```python
from build123d import *
from OCP.BRepFilletAPI import BRepFilletAPI_MakeChamfer

# Parameters (mm, degrees)
BASE_PLATE_DEPTH         = 3
INNER_START              = -3
INNER_BASE_PROFILE_DEPTH = 4
MOUNTING_START           = -7
BASEPLATE_5_R            = 1.83
MOUNTING_HOLES_DEPTH     = 7
COUNTERSINK_SIZE         = 1.7
COUNTERSINK_SIZE2        = 1.477787454


with BuildPart() as part:
    # BasePlate → Base Plate (new body)
    with BuildSketch(Plane(origin=(0, 0, 0), x_dir=(1, 0, 0), z_dir=(0, 1, 0))):
        with BuildLine():
            Line((-85, 75), (85, 75))
            ThreePointArc((85, 75), (95.606601718, 70.606601718), (100, 60))
            Line((100, 60), (100, -60))
            ThreePointArc((100, -60), (95.606601718, -70.606601718), (85, -75))
            Line((85, -75), (-85, -75))
            ThreePointArc((-85, -75), (-95.606601718, -70.606601718), (-100, -60))
            Line((-100, -60), (-100, 60))
            ThreePointArc((-100, 60), (-95.606601718, 70.606601718), (-85, 75))
        make_face()
    extrude(amount=-BASE_PLATE_DEPTH)

    # BasePlate<4> → Inner Base Profile (add)
    with BuildSketch(Plane(origin=(0, 0, 0), x_dir=(1, 0, 0), z_dir=(0, 1, 0)).offset(INNER_START)):
        with BuildLine():
            Line((-85, 73), (46, 73))
            ThreePointArc((46, 73), (47.414213562, 72.414213562), (48, 71))
            ThreePointArc((48, 71), (50, 69), (52, 71))
            ThreePointArc((52, 71), (52.585786438, 72.414213562), (54, 73))
            Line((54, 73), (85, 73))
            ThreePointArc((85, 73), (94.192388155, 69.192388155), (98, 60))
            Line((98, 60), (98, -60))
            ThreePointArc((98, -60), (94.192388155, -69.192388155), (85, -73))
            Line((85, -73), (54, -73))
            ThreePointArc((54, -73), (52.585786438, -72.414213562), (52, -71))
            ThreePointArc((52, -71), (50, -69), (48, -71))
            ThreePointArc((48, -71), (47.414213562, -72.414213562), (46, -73))
            Line((46, -73), (-85, -73))
            ThreePointArc((-85, -73), (-94.192388155, -69.192388155), (-98, -60))
            Line((-98, -60), (-98, 60))
            ThreePointArc((-98, 60), (-94.192388155, 69.192388155), (-85, 73))
        make_face()
    extrude(amount=-INNER_BASE_PROFILE_DEPTH)

    # BasePlate<5> → Mounting Holes (cut)
    with BuildSketch(Plane(origin=(0, 0, 0), x_dir=(1, 0, 0), z_dir=(0, 1, 0)).offset(MOUNTING_START)):
        with Locations(Location((90, -15, 0), (0, 0, 270))):
            Circle(BASEPLATE_5_R)
        with Locations(Location((-89, 64, 0), (0, 0, 270))):
            Circle(BASEPLATE_5_R)
        with Locations(Location((89, 64, 0), (0, 0, 270))):
            Circle(BASEPLATE_5_R)
        with Locations(Location((89, -64, 0), (0, 0, 270))):
            Circle(BASEPLATE_5_R)
        with Locations(Location((-89, -64, 0), (0, 0, 270))):
            Circle(BASEPLATE_5_R)
        with Locations(Location((0, 65, 0), (0, 0, 270))):
            Circle(BASEPLATE_5_R)
        with Locations(Location((-90, 0, 0), (0, 0, 270))):
            Circle(BASEPLATE_5_R)
        with Locations(Location((0, -65, 0), (0, 0, 270))):
            Circle(BASEPLATE_5_R)
    extrude(amount=MOUNTING_HOLES_DEPTH, mode=Mode.SUBTRACT)

    # Countersink: one chamfer whose edges measure the first distance from different faces: ONE call of the kernel's chamfer builder (chamfer() names one face for all edges)
    countersink_edges_1 = [part.edges().sort_by_distance(p)[0] for p in [
        (-89, 0, 62.17),
    ]]
    countersink_side_1 = [part.faces().sort_by_distance(p)[0] for p in [
        (-89, -3.5, 62.17),
    ]]
    countersink_edges_2 = [part.edges().sort_by_distance(p)[0] for p in [
        (0, 0, -66.83),
    ]]
    countersink_side_2 = [part.faces().sort_by_distance(p)[0] for p in [
        (0, -3.5, -66.83),
    ]]
    countersink_edges_3 = [part.edges().sort_by_distance(p)[0] for p in [
        (89, 0, -65.83),
    ]]
    countersink_side_3 = [part.faces().sort_by_distance(p)[0] for p in [
        (89, -3.5, -65.83),
    ]]
    countersink_edges_4 = [part.edges().sort_by_distance(p)[0] for p in [
        (90, 0, 13.17),
    ]]
    countersink_side_4 = [part.faces().sort_by_distance(p)[0] for p in [
        (90, -3.5, 13.17),
    ]]
    countersink_edges_5 = [part.edges().sort_by_distance(p)[0] for p in [
        (89, 0, 62.17),
    ]]
    countersink_side_5 = [part.faces().sort_by_distance(p)[0] for p in [
        (89, -3.5, 62.17),
    ]]
    countersink_edges_6 = [part.edges().sort_by_distance(p)[0] for p in [
        (-90, 0, -1.83),
    ]]
    countersink_side_6 = [part.faces().sort_by_distance(p)[0] for p in [
        (-90, -3.5, -1.83),
    ]]
    countersink_edges_7 = [part.edges().sort_by_distance(p)[0] for p in [
        (-89, 0, -65.83),
    ]]
    countersink_side_7 = [part.faces().sort_by_distance(p)[0] for p in [
        (-89, -3.5, -65.83),
    ]]
    countersink_edges_8 = [part.edges().sort_by_distance(p)[0] for p in [
        (0, 0, 63.17),
    ]]
    countersink_side_8 = [part.faces().sort_by_distance(p)[0] for p in [
        (0, -3.5, 63.17),
    ]]
    countersink = BRepFilletAPI_MakeChamfer(part.part.solid().wrapped)
    for e in countersink_edges_1:
        countersink.Add(COUNTERSINK_SIZE, COUNTERSINK_SIZE2, e.wrapped, countersink_side_1[0].wrapped)  # the first distance lies on this face
    for e in countersink_edges_2:
        countersink.Add(COUNTERSINK_SIZE, COUNTERSINK_SIZE2, e.wrapped, countersink_side_2[0].wrapped)  # the first distance lies on this face
    for e in countersink_edges_3:
        countersink.Add(COUNTERSINK_SIZE, COUNTERSINK_SIZE2, e.wrapped, countersink_side_3[0].wrapped)  # the first distance lies on this face
    for e in countersink_edges_4:
        countersink.Add(COUNTERSINK_SIZE, COUNTERSINK_SIZE2, e.wrapped, countersink_side_4[0].wrapped)  # the first distance lies on this face
    for e in countersink_edges_5:
        countersink.Add(COUNTERSINK_SIZE, COUNTERSINK_SIZE2, e.wrapped, countersink_side_5[0].wrapped)  # the first distance lies on this face
    for e in countersink_edges_6:
        countersink.Add(COUNTERSINK_SIZE, COUNTERSINK_SIZE2, e.wrapped, countersink_side_6[0].wrapped)  # the first distance lies on this face
    for e in countersink_edges_7:
        countersink.Add(COUNTERSINK_SIZE, COUNTERSINK_SIZE2, e.wrapped, countersink_side_7[0].wrapped)  # the first distance lies on this face
    for e in countersink_edges_8:
        countersink.Add(COUNTERSINK_SIZE, COUNTERSINK_SIZE2, e.wrapped, countersink_side_8[0].wrapped)  # the first distance lies on this face
    add(Compound.cast(countersink.Shape()), mode=Mode.REPLACE)


solid = part.part
```
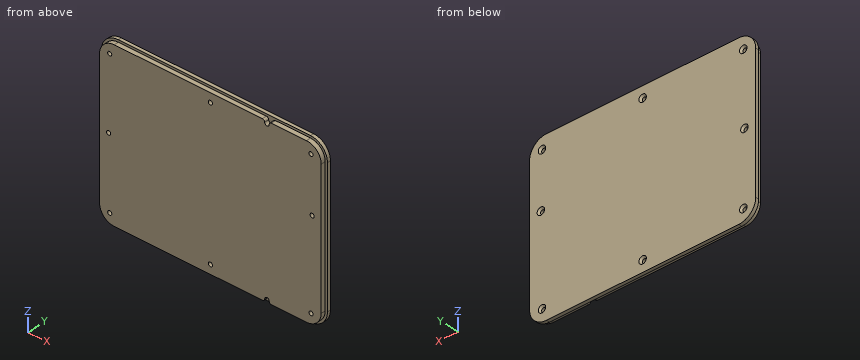
Verification items for the finished model (mm, model axes). Give positions to 0.01 mm unless a question says otherwise; leave off trailing zeros. Loops run counter-clockwise (first coordinate to the right, second up) from the corner with the lowest first, then second, coordinate; pieces in that order, holes last. Notation, with made-up numbers: M -39,36.25 L -7,36.25 A20 ccw -7,41.25 Z; hole C 45,48.5 d9. An arc over 180 degrees is marked long. Return JSON: item names as keys, results as strings.
1) Section check B-B, the plane x = 10.5. Enter the section's corners in (y, z), and give its area (3 significant figures).
Findings:
{"outline": "M -7,-73 L -3,-73 L -3,-75 L 0,-75 L 0,75 L -3,75 L -3,73 L -7,73 Z", "area": "1,030 mm2"}
2) Gauge pin test, flat ends, axial feed: P1, Ø3, axis at x = 90, z = 15, coming from the -Y side; P2, Ø3, axis at x = 71.5, y = -5, coming from the -Z side; P3, Ø3, axis at x = 65.5, y = -5, coming from the +Z side; P4, Ø1.2, axis at y = -5, z = -25.5, coming from the +X side. Record the tip position at first contact, or that the pin passes through.
Findings:
{"P1": "passes through", "P2": "stops at z = -73", "P3": "stops at z = 73", "P4": "stops at x = 98"}
3) Section check A-A, the plane y = -4.5. Count the separate pieces of the cut face and the enclosed holes in it, and give its area (3 significant figures).
Findings:
{"separate pieces": "1", "enclosed holes": "8", "area": "28,400 mm2"}
4) Material ranges on L1, parallel to X at y = -1, z = -62.5; L2, parallel to X at y = -4.6, z = 64; L3, parallel to Z at x = 89, y = -5.2, recorded low to high. Write a range as [from, to].
Findings:
{"L1": "x = [-99.79, -90.92], [-87.08, 87.08], [90.92, 99.79]", "L2": "x = [-97.37, -90.83], [-87.17, -1.53], [1.53, 87.17], [90.83, 97.37]", "L3": "z = [-72.37, -65.83], [-62.17, 13.47], [16.53, 62.17], [65.83, 72.37]"}
